Solid Edge part; units mm, degrees
sketch "Sketch1" plane through (0, 0, 0) normal (1, 0, 0) x (0, 1, 0)
  circle A0 centre (0, 0) radius 2.5
extrude "Protrusion1" add sketch "Sketch1" along normal mid plane 80
sketch "Sketch2" plane through (40, 0, 0) normal (1, 0, 0) x (0, 1, 0)
  circle A0 centre (0, 0) radius 2
extrude "Extrusionsausschnitt_1" cut sketch "Sketch2" against normal blind 10 flip side to cut
cosmetic_thread "Thread1"
chamfer "Fase_1" distance 0.5 angle 45 1 edges at (40, -2, 0)
sketch "Sketch3" plane through (-40, 0, 0) normal (-1, 0, 0) x (0, 0, 1)
  circle A0 centre (0, 0) radius 2
extrude "Extrusionsausschnitt_2" cut sketch "Sketch3" against normal blind 10 flip side to cut
cosmetic_thread "Thread2"
properties material "Aluminiumlegierung:3.0205, Al 99.0, EN-AW 1200"
Could you check a few things on this model? Use its own coordinates, in mm. A direction names the side the tool comes from. Give positions to 0.01 mm unless a question says otherwise; leave off trailing zeros. Write each loop counter-clockwise with the first axis right and the second up, starting at its lowest first coordinate (ties: lowest second). Pieces come first, ordered by that corner, then holes. Notation, with made-up numbers: (72, -24.75) -> (114, -24.75) arc R19 cw to (114, 3.25) -> close; hole circle Ø10 at (42.25, 1.5). An arc over 180 degrees is marked (long way). Write each question's results on one line, items separated by ' | '. Start each with the question number.
Q1. Which directions (+Z, -Z, +X, -X, +Y, -Y) give clear straight access to the entire face, cutting with the end or side of a thin tool? Please do faces 1 (the face through (-40, 0, 0)), 2 (the face through (-30, -2, 1)), 3 (the face through (35, 0, -2)).
Q2. Suppose I cut it at A-A, the plane z = 0. List the corners of the cut face in (x, y) for me, and give its area (3 significant figures).
Q3. We'd pull the mould along Z, two halves only. Please class faces 4 (the face through (-35, -2, 0)), 5 (the face through (40, 0, 0)): +Z half, -Z half, draft (parallel to the pull), parting line (faces both ways), or undercut.
Q4. I need wall thicknesses on probe 1 along X at (y, z) = (-1.7, -1.8); probe 2 along Z at (x, y) = (-11, -2). Which ranges of each line are inside material? Lowest first, please.
Q5. I'm going to push flat-ended pins straight in: pin 1 Ø1 at (x, z) = (-30, 1) entering from +Y; pin 2 Ø1 at (x, y) = (-25.5, -1) entering from +Z. Where does each tip first touch, or does it pass through?
Q6. Suppose I cut it at C-C, the plane x = -22. List the corners of the cut face in (y, z) for me, and give its area (3 significant figures).
Outcome:
1) face 1: +Z, -Z, -X, +Y, -Y | face 2: -X | face 3: +X
2) outline: (-40, -2) -> (-30, -2) -> (-30, -2.5) -> (30, -2.5) -> (30, -2) -> (39.5, -2) -> (40, -1.5) -> (40, 1.5) -> (39.5, 2) -> (30, 2) -> (30, 2.5) -> (-30, 2.5) -> (-30, 2) -> (-40, 2) -> close | area: 380 mm2
3) face 4: parting line | face 5: draft
4) probe 1: -30 to 30 | probe 2: -1.5 to 1.5
5) pin 1: y = 2.45 | pin 2: z = 2.45
6) outline: circle Ø5 at (0, 0) | area: 19.6 mm2
